from build123d import *

# Parameters (mm, degrees)
SKETCH1_W           = 60
SKETCH1_H           = 60
BOSS_EXTRUDE1_DEPTH = 2
SKETCH2_R           = 2
CUT_EXTRUDE1_DEPTH  = 3
SKETCH3_W           = 21
SKETCH3_H           = 15
CUT_EXTRUDE2_DEPTH  = 2


with BuildPart() as part:
    # Sketch1 → Boss-Extrude1 (new body)
    with BuildSketch(Plane(origin=(0, 0, 0), x_dir=(1, 0, 0), z_dir=(0, 1, 0))):
        Rectangle(SKETCH1_W, SKETCH1_H)
    extrude(amount=BOSS_EXTRUDE1_DEPTH)

    # Sketch2 → Cut-Extrude1 (cut, through all)
    with BuildSketch(Plane(origin=(0, 2, 0), x_dir=(1, 0, 0), z_dir=(0, 1, 0))):
        with Locations((-26, 26)):
            Circle(SKETCH2_R)
        with Locations((0, 26)):
            Circle(SKETCH2_R)
        with Locations((26, 26)):
            Circle(SKETCH2_R)
        with Locations((26, -26)):
            Circle(SKETCH2_R)
        with Locations((0, -26)):
            Circle(SKETCH2_R)
        with Locations((-26, -26)):
            Circle(SKETCH2_R)
    extrude(amount=-CUT_EXTRUDE1_DEPTH, mode=Mode.SUBTRACT)

    # Sketch3 → Cut-Extrude2 (cut)
    with BuildSketch(Plane(origin=(0, 2, 0), x_dir=(1, 0, 0), z_dir=(0, 1, 0))):
        Rectangle(SKETCH3_W, SKETCH3_H)
    extrude(amount=-CUT_EXTRUDE2_DEPTH, mode=Mode.SUBTRACT)


solid = part.part
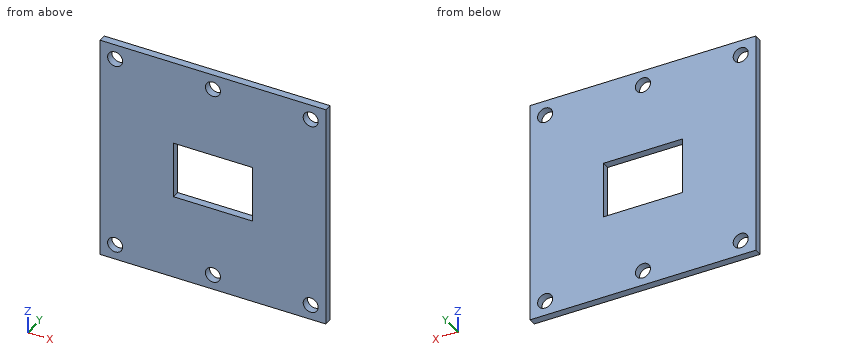
Design review of the part built by this model. Coordinates are the model's own, in mm. Round coordinates to 2 decimals unless told otherwise and drop trailing zeros. Loops run counter-clockwise (first coordinate to the right, second up) from the corner with the lowest first, then second, coordinate; pieces in that order, holes last. Notation, with made-up numbers: M 78.25,53.5 L 104.25,53.5 A16 ccw 104.25,70.5 Z; hole C 12.25,55 d2. An arc over 180 degrees is marked long. Answer as a JSON object with one key per item and string values.
Item 1: We need section D-D on x = 26. Give the boundary of the cut face in (y, z), and give its area (3 significant figures).
Answer sheet:
{"outline": "M 0,-30 L 2,-30 L 2,-28 L 0,-28 Z; M 0,-24 L 2,-24 L 2,24 L 0,24 Z; M 0,28 L 2,28 L 2,30 L 0,30 Z", "area": "104 mm^2"}
Item 2: Wall thickness on L1, parallel to Z at x = 26, y = 1.15; L2, parallel to X at y = 1.1, z = -26; L3, parallel to Z at x = 0, y = 1.6: over which ranges is each line inside the solid? List them lowest first. Write a range as from..to.
Answer sheet:
{"L1": "z = -30..-28, -24..24, 28..30", "L2": "x = -30..-28, -24..-2, 2..24, 28..30", "L3": "z = -30..-28, -24..-7.5, 7.5..24, 28..30"}
Item 3: We need section B-B on y = 0.4. Give the boundary of the cut face in (x, z), and give its area (3 significant figures).
Answer sheet:
{"outline": "M -30,-30 L 30,-30 L 30,30 L -30,30 Z; hole C -26,-26 d4; hole C -26,26 d4; hole M -10.5,-7.5 L 10.5,-7.5 L 10.5,7.5 L -10.5,7.5 Z; hole C 0,-26 d4; hole C 0,26 d4; hole C 26,-26 d4; hole C 26,26 d4", "area": "3,210 mm^2"}
Item 4: We need section C-C on z = -4. Give the boundary of the cut face in (x, y), and give its area (3 significant figures).
Answer sheet:
{"outline": "M -30,0 L -10.5,0 L -10.5,2 L -30,2 Z; M 10.5,0 L 30,0 L 30,2 L 10.5,2 Z", "area": "78.0 mm^2"}
Item 5: We need section A-A on x = 0. Give the boundary of the cut face in (y, z), and give its area (3 significant figures).
Answer sheet:
{"outline": "M 0,-30 L 2,-30 L 2,-28 L 0,-28 Z; M 0,-24 L 2,-24 L 2,-7.5 L 0,-7.5 Z; M 0,7.5 L 2,7.5 L 2,24 L 0,24 Z; M 0,28 L 2,28 L 2,30 L 0,30 Z", "area": "74.0 mm^2"}
